Here's the drawing with two shaded views (mm, measured from the low corner). I have some questions. Round coordinates to 2 decimals unless told otherwise and drop trailing zeros. Loops run counter-clockwise (first coordinate to the right, second up) from the corner with the lowest first, then second, coordinate; pieces in that order, holes last. Notation, with made-up numbers: M 81,51 L 127,51 A27 cw 127,79 Z; hole C 6,-22 d6. An arc over 180 degrees is marked long. Answer as a JSON object with one key per item and string values.
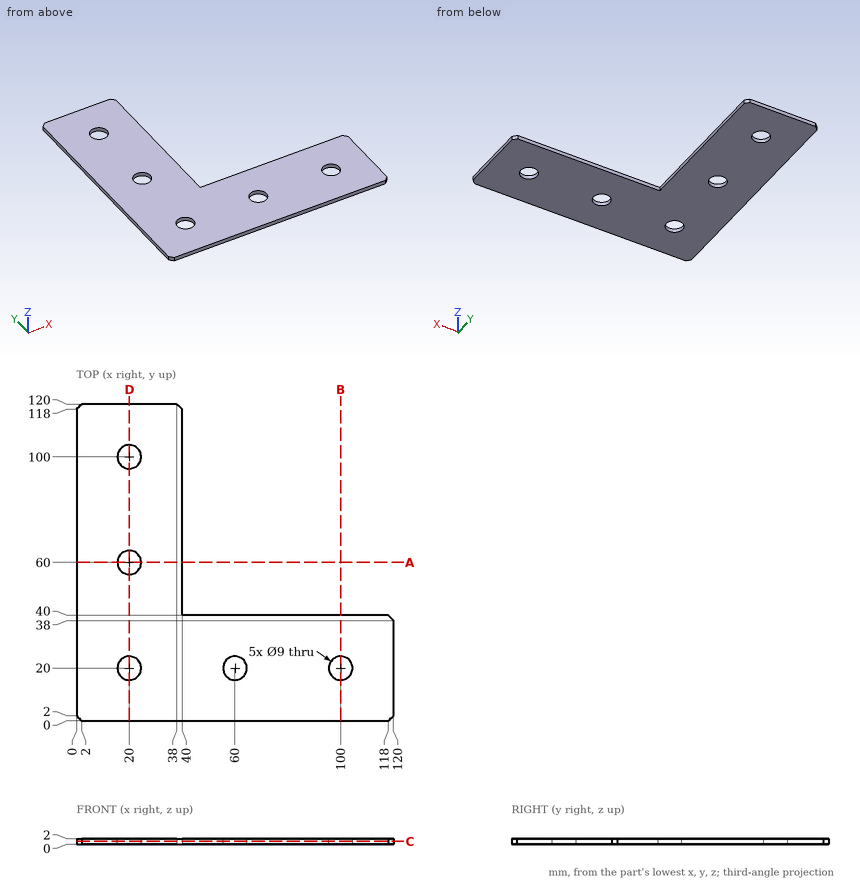
Item 1: If I drill on L1, parallel to X at y = 20, z = 1.3; L2, parallel to Y at x = 19.5, z = 0.9; L3, parallel to Y at x = 60, z = 0.6, over which ranges is the centre line in solid material (lowest first)? Write a range as from..to.
Solution:
{"L1": "x = 0..15.5, 24.5..55.5, 64.5..95.5, 104.5..120", "L2": "y = 0..15.53, 24.47..55.53, 64.47..95.53, 104.47..120", "L3": "y = 0..15.5, 24.5..40"}
Item 2: I want a section at D-D on x = 20. List the corners of the cut face in (y, z) for me.
Solution:
{"outline": "M 0,0 L 15.5,0 L 15.5,2 L 0,2 Z; M 24.5,0 L 55.5,0 L 55.5,2 L 24.5,2 Z; M 64.5,0 L 95.5,0 L 95.5,2 L 64.5,2 Z; M 104.5,0 L 120,0 L 120,2 L 104.5,2 Z"}
Item 3: I want a section at C-C on z = 1.1. List the corners of the cut face in (x, y) for me, plus the area to 3 significant figures.
Solution:
{"outline": "M 0,2 L 2,0 L 118,0 L 120,2 L 120,38 L 118,40 L 40,40 L 40,118 L 38,120 L 2,120 L 0,118 Z; hole C 20,20 d9; hole C 20,60 d9; hole C 20,100 d9; hole C 60,20 d9; hole C 100,20 d9", "area": "7,670 mm2"}
Item 4: I want a section at A-A on y = 60. List the corners of the cut face in (x, z) for me, plus the area to 3 significant figures.
Solution:
{"outline": "M 0,0 L 15.5,0 L 15.5,2 L 0,2 Z; M 24.5,0 L 40,0 L 40,2 L 24.5,2 Z", "area": "62.0 mm2"}
Item 5: For P1, Ø7, axis at x = 100, y = 20, coming from the -Z side, with a flat end and sliding along its axis, tell me the tip position at first contact or that it passes through.
Solution:
{"P1": "passes through"}
